Build history of the part. All positions in model axes, mm. Face numbers are marked on the shaded views. Coordinates: 2 decimals unless noted, no trailing zeros. Order: outer loops, then holes, each group sorted by start corner. A loop starts at its lowest first (then second) coordinate and runs counter-clockwise, first axis right, second up. Notation, with made-up numbers: (21, 46) - (27, 46) arc R28 ccw to (27, 66) - close; hole circle Ø8 at (85.5, 31.5). An arc over 180 degrees is marked (long way). Return JSON: item names as keys, results as strings.
Autodesk Inventor part; units mm, degrees
ref_plane "YZ Plane" through (0, 0, 0) normal (1, 0, 0) x (0, 1, 0)
ref_plane "XZ Plane" through (0, 0, 0) normal (0, 1, 0) x (-1, 0, 0)
ref_plane "XY Plane" through (0, 0, 0) normal (0, 0, 1) x (1, 0, 0)
sketch "Sketch1" plane through (0, 0, 0) normal (1, 0, 0) x (0, 1, 0)
  line L0 (12.7, 19.05) -> (-12.7, 19.05)
  line L1 (-12.7, 19.05) -> (-12.7, -19.05)
  line L2 (-12.7, -19.05) -> (12.7, -19.05)
  line L3 (12.7, -19.05) -> (12.7, 19.05)
  line L4 (12.7, 19.05) -> (-12.7, -19.05) construction
  line L5 (-12.7, 19.05) -> (12.7, -19.05) construction
  arc A0 (6.0166, 15.4771) -> (9.2234, 15.4771) centre (7.62, 12.7) ccw
  line L6 (6.0166, 15.4771) -> (9.2234, 15.4771)
  arc A1 (6.0008, 2.8046) -> (9.2393, 2.8046) centre (7.62, 0) ccw
  line L7 (6.0008, 2.8046) -> (9.2393, 2.8046)
  arc A2 (5.969, -9.8404) -> (9.271, -9.8404) centre (7.62, -12.7) ccw
  line L8 (5.969, -9.8404) -> (9.271, -9.8404)
  arc A3 (-9.3345, 15.6696) -> (-5.9055, 15.6696) centre (-7.62, 12.7) ccw
  line L9 (-9.3345, 15.6696) -> (-5.9055, 15.6696)
  arc A4 (-9.398, 3.0796) -> (-5.842, 3.0796) centre (-7.62, 0) ccw
  line L10 (-9.398, 3.0796) -> (-5.842, 3.0796)
  arc A5 (-9.4456, -9.5379) -> (-5.7944, -9.5379) centre (-7.62, -12.7) ccw
  line L11 (-9.4456, -9.5379) -> (-5.7944, -9.5379)
  line L12 (3.4886, 13.1373) -> (1.0834, 13.1373)
  line L13 (1.0834, 13.1373) -> (1.0834, 12.2627)
  line L14 (1.0834, 12.2627) -> (3.4886, 12.2627)
  line L15 (3.4886, 12.2627) -> (3.4886, 13.1373)
  line L16 (3.4886, 13.1373) -> (1.0834, 12.2627) construction
  line L17 (1.0834, 13.1373) -> (3.4886, 12.2627) construction
  line L18 (12.7, 0) -> (-12.7, 0) construction
  line L19 (3.4886, 1.3826) -> (1.0834, 1.3826)
  line L20 (1.0834, 1.3826) -> (1.0834, 0.508)
  line L21 (1.0834, 0.508) -> (3.4886, 0.508)
  line L22 (3.4886, 0.508) -> (3.4886, 1.3826)
  line L23 (3.4886, 1.3826) -> (1.0834, 0.508) construction
  line L24 (1.0834, 1.3826) -> (3.4886, 0.508) construction
  line L25 (3.4886, -0.508) -> (1.0834, -0.508)
  line L26 (1.0834, -0.508) -> (1.0834, -1.3826)
  line L27 (1.0834, -1.3826) -> (3.4886, -1.3826)
  line L28 (3.4886, -1.3826) -> (3.4886, -0.508)
  line L29 (3.4886, -0.508) -> (1.0834, -1.3826) construction
  line L30 (1.0834, -0.508) -> (3.4886, -1.3826) construction
  line L31 (1.0834, -13.1373) -> (3.4886, -13.1373)
  line L32 (3.4886, -12.2627) -> (1.0834, -12.2627)
  line L33 (1.0834, -12.2627) -> (1.0834, -13.1373)
  line L34 (3.4886, -13.1373) -> (3.4886, -12.2627)
  line L35 (3.4886, -12.2627) -> (1.0834, -13.1373) construction
  line L36 (1.0834, -12.2627) -> (3.4886, -13.1373) construction
  line L37 (1.0834, -15.0279) -> (3.4886, -15.0279)
  line L38 (3.4886, -14.1533) -> (1.0834, -14.1533)
  line L39 (1.0834, -14.1533) -> (1.0834, -15.0279)
  line L40 (3.4886, -15.0279) -> (3.4886, -14.1533)
  line L41 (3.4886, -14.1533) -> (1.0834, -15.0279) construction
  line L42 (1.0834, -14.1533) -> (3.4886, -15.0279) construction
  line L43 (3.4886, -10.3721) -> (1.0834, -10.3721)
  line L44 (1.0834, -10.3721) -> (1.0834, -11.2467)
  line L45 (1.0834, -11.2467) -> (3.4886, -11.2467)
  line L46 (3.4886, -11.2467) -> (3.4886, -10.3721)
  line L47 (3.4886, -10.3721) -> (1.0834, -11.2467) construction
  line L48 (1.0834, -10.3721) -> (3.4886, -11.2467) construction
  line L49 (-0.889, 13.97) -> (-0.889, 11.43)
  line L50 (-0.889, 11.43) -> (-3.0887, 12.7)
  line L51 (-3.0887, 12.7) -> (-0.889, 13.97)
  circle A6 centre (-1.905, 0) radius 1.27
  arc A7 (-1.905, -15.0279) -> (-1.905, -10.3721) centre (-3.4035, -12.7) ccw
  line L52 (-1.905, -10.3721) -> (-1.905, -15.0279)
  point P0 (0, 0)
  point P1 (2.286, 12.7)
  point P2 (0, 19.05)
  point P3 (2.286, 0.9453)
  point P4 (2.286, -0.9453)
  point P5 (2.286, -12.7)
  point P6 (2.286, -14.5906)
  point P7 (2.286, -10.8094)
  point P8 (2.286, -12.2627)
  point P9 (2.286, -11.2467)
  point P10 (-0.889, 12.7)
  point P11 (0, 0)
  dimension "d0" = 6.4135
  dimension "d1" = 3.2067
  dimension "d2" = 6.477
  dimension "d3" = 3.2385
  dimension "d4" = 6.604
  dimension "d5" = 3.302
  dimension "d6" = 6.858
  dimension "d7" = 3.429
  dimension "d8" = 7.112
  dimension "d9" = 3.556
  dimension "d10" = 7.3025
  dimension "d11" = 3.6513
  dimension "d12" = 38.1
  dimension "d13" = 6.35
  dimension "d14" = 6.35
  dimension "d15" = 5.08
  dimension "d16" = 25.4
  dimension "d17" = 5.08
  dimension "d18" = 0.8746
  dimension "d19" = 2.4052
  dimension "d20" = 2.286
  dimension "d21" = 0.8746
  dimension "d22" = 2.4052
  dimension "d23" = 0.8746
  dimension "d24" = 2.4052
  dimension "d25" = 0.508
  dimension "d26" = 0.508
  dimension "d27" = 0.8746
  dimension "d28" = 2.4052
  dimension "d29" = 0.8746
  dimension "d30" = 2.4052
  dimension "d31" = 0.8746
  dimension "d32" = 2.4052
  dimension "d33" = 1.016
  dimension "d35" = 1.016
  dimension "d36" = 2.54
  dimension "d38" = 2.54
  dimension "d39" = 2.54
  dimension "d40" = 0.889
  dimension "d41" = 2.54
  dimension "d42" = 1.905
  dimension "d43" = 4.6558
  dimension "d44" = 2.7685
  dimension "d45" = 5.6895
  dimension "d46" = 6.35
extrude "Extrusion1" add sketch "Sketch1" along normal blind 10
extrude "Extrusion2" add sketch "Sketch1" along normal blind 11 contours L15 L14 L13 L12 | L22 L21 L20 L19 | L28 L27 L26 L25 | L33 L32 L34 L31 | L39 L38 L40 L37 | L46 L45 L44 L43 | L49 L50 L51 | A6 | L52 A7
equation "\"d38\" = d36"
equation "\"d39\" = d36"
properties part number "shaft hole tester"
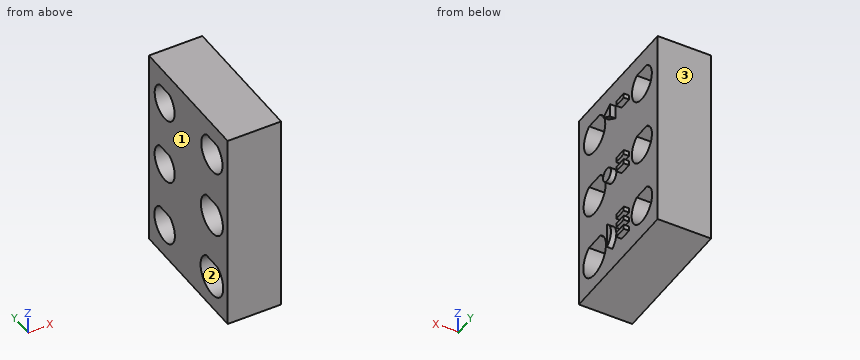
1. Cut at C-C on x = 2.25. Give the cut face in (y, z), plus the area to 3 significant figures.
Check values:
{"outline": "(-12.7, -19.05) - (12.7, -19.05) - (12.7, 19.05) - (-12.7, 19.05) - close; hole (-9.45, -9.54) arc R3.65 ccw (long way) to (-5.79, -9.54) - close; hole (-9.4, 3.08) arc R3.56 ccw (long way) to (-5.84, 3.08) - close; hole (-9.33, 15.67) arc R3.43 ccw (long way) to (-5.91, 15.67) - close; hole (5.97, -9.84) arc R3.3 ccw (long way) to (9.27, -9.84) - close; hole (6, 2.8) arc R3.24 ccw (long way) to (9.24, 2.8) - close; hole (6.02, 15.48) arc R3.21 ccw (long way) to (9.22, 15.48) - close", "area": "756 mm²"}
2. Cut at B-B on y = -7.62. Give the cut face in (x, z), plus the area to 3 significant figures.
Check values:
{"outline": "(0, -19.05) - (10, -19.05) - (10, -16.35) - (0, -16.35) - close; (0, -9.54) - (10, -9.54) - (10, -3.56) - (0, -3.56) - close; (0, 3.08) - (10, 3.08) - (10, 9.27) - (0, 9.27) - close; (0, 15.67) - (10, 15.67) - (10, 19.05) - (0, 19.05) - close", "area": "183 mm²"}
3. Probe L1, parallel to Y at x = 6.25, z = -12.7; L2, parallel to Z at x = 5.75, y = 7.5; L3, parallel to Y at x = 4, z = 12.7. List the from-to ranges inside material, lowest first.
Check values:
{"L1": "-12.7 to -11.27, -3.97 to 4.32, 10.92 to 12.7", "L2": "-19.05 to -16, -9.84 to -3.24, 2.8 to 9.5, 15.48 to 19.05", "L3": "-12.7 to -11.05, -4.19 to 4.41, 10.83 to 12.7"}
4. Drop flat-ended pins along their axis: pin 1 (1.5 mm diameter, centred on y = -6, z = 6, fed in from +X); pin 2 (0.8 mm diameter, centred on x = 10.5, y = 2.5, fed in from -Z); pin 3 (0.5 mm diameter, centred on x = 10.5, y = 2, fed in from +Z). Give the stop position or say it passes through.
Check values:
{"pin 1": "x = 10", "pin 2": "z = -15.03", "pin 3": "z = 13.14"}
5. Mould opens along Y. For the marked faces 1, 2 and 3 say: pulls with the +Y half, pulls with the -Y half, needs draft (parallel to the pull), parting line crosses it, or undercut.
Check values:
{"face 1": "needs draft", "face 2": "undercut", "face 3": "pulls with the +Y half"}
6. Cut at D-D on z = 0. Give the cut face in (x, y) (3 decimals), plus the area to 3 significant figures.
Check values:
{"outline": "(0, -12.7) - (10, -12.7) - (10, -11.176) - (0, -11.176) - close; (0, -4.064) - (10, -4.064) - (10, -3.175) - (11, -3.175) - (11, -0.635) - (10, -0.635) - (10, 4.382) - (0, 4.382) - close; (0, 10.859) - (10, 10.859) - (10, 12.7) - (0, 12.7) - close", "area": "121 mm²"}
7. Cut at A-A on z = -12.7. Give the cut face in (x, y) (3 decimals), plus the area to 3 significant figures.
Check values:
{"outline": "(0, -12.7) - (10, -12.7) - (10, -11.271) - (0, -11.271) - close; (0, -3.969) - (10, -3.969) - (10, -1.905) - (11, -1.905) - (11, -0.635) - (10, -0.635) - (10, 1.083) - (11, 1.083) - (11, 3.489) - (10, 3.489) - (10, 4.318) - (0, 4.318) - close; (0, 10.922) - (10, 10.922) - (10, 12.7) - (0, 12.7) - close", "area": "119 mm²"}
